from build123d import *

# Parameters (mm, degrees)
BOSS_EXTRUDE1_DEPTH = 400
SKETCH3_R           = 125
BOSS_EXTRUDE2_DEPTH = 500
FILLET1_R           = 100
SKETCH5_R           = 125
CUT_EXTRUDE1_DEPTH  = 2046


with BuildPart() as part:
    # Sketch1 → Boss-Extrude1 (new body)
    with BuildSketch(Plane.XY):
        with BuildLine():
            Line((15.274151436, 50), (15.274151436, 700))
            ThreePointArc((15.274151436, 700), (65.274151436, 750), (115.274151436, 700))
            Line((115.274151436, 700), (115.274151436, -50))
            Line((115.274151436, -50), (-784.725848564, -50))
            Line((-784.725848564, -50), (-784.725848564, 700))
            ThreePointArc((-784.725848564, 700), (-734.725848564, 750), (-684.725848564, 700))
            Line((-684.725848564, 700), (-684.725848564, 50))
            Line((-684.725848564, 50), (15.274151436, 50))
        make_face()
    extrude(amount=BOSS_EXTRUDE1_DEPTH)

    # Sketch3 → Boss-Extrude2 (add)
    with BuildSketch(Plane.XZ.offset(50)):
        with Locations(Location((-334.725848564, 200, 0), (0, 0, 270))):
            Circle(SKETCH3_R)
    extrude(amount=BOSS_EXTRUDE2_DEPTH)

    # Fillet1
    fillet1_edges = [part.edges().sort_by_distance(p)[0] for p in [
        (15.274151436, 50, 200),
        (115.274151436, -50, 200),
        (-784.725848564, -50, 200),
        (-684.725848564, 50, 200),
    ]]
    fillet(fillet1_edges, radius=FILLET1_R)

    # Sketch5 → Cut-Extrude1 (cut)
    with BuildSketch(Plane.ZY.offset(784.725848564)):
        with Locations(Location((200, 550, 0), (0, 0, 90))):
            Circle(SKETCH5_R)
    extrude(amount=-CUT_EXTRUDE1_DEPTH, mode=Mode.SUBTRACT)


solid = part.part
Model file for the job. Use its own axes, mm. A direction names the side the tool comes from. Coordinates: 2 decimals unless noted, no trailing zeros. Write each loop counter-clockwise with the first axis right and the second up, starting at its lowest first coordinate (ties: lowest second). Pieces come first, ordered by that corner, then holes. Notation, with made-up numbers: (41, 46) - (56, 46) arc R24 ccw to (56, 72) - close; hole circle Ø1 at (74, -3.5). An arc over 180 degrees is marked (long way). Write each question's results on one line, items separated by ' | '. Start each with the question number.
1) Cut at C-C (y = 364.5). Write the cut outline in (x, z).
2) Flat gauge pins, fed straight in: P1, Ø8, axis at y = -258, z = 117, coming from the +X side; P2, Ø2, axis at y = -23, z = 77, coming from the -X side; P3, Ø2, axis at x = -555.5, z = 236.5, coming from the -Y side. Where does each tip first touch, or does it go through?
3) Cut at A-A (z = 200). Write the cut outline in (x, y), then the cut area to 3 significant figures.
4) Cut at B-B (y = 550). Write the cut outline in (x, z).
5) 3-axis set-ups, long thin cutter, end or side, ignore diameter. For faces 4 (the face through (-333, -550, 202)), 5 (the face through (-210.79, -296.5, 216.27)), 6 (the face through (-13.242, 80.071, 202.8)): which of +Z, -Z, +X, -X, +Y, -Y reach the whole face in a straight line?
6) Probe line 1 along Z through (x, y) = (63.5, 550); line 2 along X through (y, z) = (369, 263.5); line 3 along Y through (x, z) = (-373, 331). List the from-to ranges inside material, lowest first. Write a range as from..to.
7) Mould opens along X. For faces 1 (the face through (-735.426, 607.68, 310.896)), 2 (the face through (115.274, 380, 197)), 3 (the face through (-735.825, 749.988, 197.2)) say: pulls with the +X half, pulls with the -X half, needs draft (parallel to the pull), parting line crosses it, or undercut.
8) Cut at D-D (x = -288). Write the cut outline in (y, z).
Returned:
1) outline: (-784.73, 0) - (-684.73, 0) - (-684.73, 400) - (-784.73, 400) - close; (15.27, 0) - (115.27, 0) - (115.27, 400) - (15.27, 400) - close
2) P1: x = -237.85 | P2: x = -754.12 | P3: y = -50
3) outline: (-784.73, 50) arc R100 ccw to (-684.73, -50) - (-459.73, -50) - (-459.73, -550) - (-209.73, -550) - (-209.73, -50) - (15.27, -50) arc R100 ccw to (115.27, 50) - (115.27, 425) - (15.27, 425) - (15.27, 150) arc R100 cw to (-84.73, 50) - (-584.73, 50) arc R100 cw to (-684.73, 150) - (-684.73, 425) - (-784.73, 425) - close; (-784.73, 675) - (-684.73, 675) - (-684.73, 700) arc R50 ccw to (-784.73, 700) - close; (15.27, 675) - (115.27, 675) - (115.27, 700) arc R50 ccw to (15.27, 700) - close | area: 303,000 mm^2
4) outline: (-784.73, 0) - (-684.73, 0) - (-684.73, 75) - (-784.73, 75) - close; (-784.73, 325) - (-684.73, 325) - (-684.73, 400) - (-784.73, 400) - close; (15.27, 0) - (115.27, 0) - (115.27, 75) - (15.27, 75) - close; (15.27, 325) - (115.27, 325) - (115.27, 400) - (15.27, 400) - close
5) face 4: +Z, -Z, +X, -X, -Y | face 5: -Y | face 6: +Z, -Z, +Y
6) line 1: 0..75, 325..400 | line 2: -784.73..-684.73, 15.27..115.27 | line 3: -50..50
7) face 1: needs draft | face 2: pulls with the +X half | face 3: undercut
8) outline: (-550, 84.06) - (-50, 84.06) - (-50, 0) - (50, 0) - (50, 400) - (-50, 400) - (-50, 315.94) - (-550, 315.94) - close
